The listing builds one solid part. Answer for the finished solid, in the listing's coordinates (mm). Coordinates: 2 decimals unless noted, no trailing zeros. Loops run counter-clockwise (first coordinate to the right, second up) from the corner with the lowest first, then second, coordinate; pieces in that order, holes last. Notation, with made-up numbers: (8.25, 53) - (15.25, 53) arc R28 cw to (15.25, 77) - close; hole circle Ø6 at (-23.75, 74.25). An arc over 180 degrees is marked (long way). One line per question, with ' | ' between items.
Autodesk Inventor part; units mm, degrees
ref_plane "Work Plane1" through (29, 0, 0) normal (0, -1, 0) x (1, 0, 0)
ref_plane "YZ Plane" through (0, 0, 0) normal (1, 0, 0) x (0, 1, 0)
ref_plane "XZ Plane" through (0, 0, 0) normal (0, 1, 0) x (-1, 0, 0)
sketch "Sketch1" plane through (0, 0, 0) normal (0, 0, 1) x (1, 0, 0)
  line L0 (-0.0833, 0) -> (35, 0)
  line L1 (35, 0) -> (35, 1)
  line L2 (35, 1) -> (32, 1)
  line L3 (32, 1) -> (31.6932, 1)
  line L4 (31.6932, 1) -> (0, 1)
  line L5 (0, 1) -> (0, 1.75)
  line L6 (0, 1.75) -> (-1.2, 1.75)
  line L7 (-1.2, 1.75) -> (-1.2, 0.7217)
  line L8 (-1.2, 0.7217) -> (-0.5, 0.7217)
  line L9 (-0.5, 0.7217) -> (-0.0833, 0)
  line L10 (-8.44, 0) -> (42.24, 0)
  line L11 (0, -0.35) -> (0, 2.1)
  line L12 (32, 1) -> (0, 1) construction
  dimension "d1" = 3
  dimension "d2" = 0.3068
  dimension "d3" = 1.2
  dimension "d4" = 0.7
  dimension "d5" = 60
  dimension "d6" = 2
  dimension "d7" = 2
  dimension "d8" = 1.4434
  dimension "d9" = 3.5
  dimension "d26" = 35
revolve "Body" add sketch "Sketch1" angle 360 about axis through (-0.0833, 0, 0) along (1, 0, 0)
sketch "Sketch2" plane through (-1.2, 0, 0) normal (-1, 0, 0) x (0, 0, 1)
  circle A0 centre (0, 0) radius 0.7217
  line L0 (0, -2.45) -> (0, 2.45)
  line L1 (-2.45, 0) -> (2.45, 0)
  line L2 (0.7217, 0) -> (0.3608, -0.625)
  line L3 (0.3608, -0.625) -> (-0.3608, -0.625)
  line L4 (-0.3608, -0.625) -> (-0.7217, 0)
  line L5 (-0.7217, 0) -> (-0.3608, 0.625)
  line L6 (-0.3608, 0.625) -> (0.3608, 0.625)
  line L7 (0.3608, 0.625) -> (0.7217, 0)
extrude "Slot" add sketch "Sketch2" against normal up to next contours L7 A0 | A0 L2 | L6 L0 A0 | A0 L0 L3 | L0 L6 A0 | A0 L3 L0 | L4 A0 | A0 L5
fillet "Fillet1" radius 0.8 1 edges at (-1.2, -1.75, 0)
chamfer "Chamfer1" distance 0.3067 distance2 0.3067 1 edges at (35, -1, 0) measured on face at (35, 0.3333, 0.4421)
ref_plane "Work Plane1" through (29, 0, 0) normal (0, -1, 0) x (1, 0, 0)
fillet "Fillet2" radius 0.1 1 edges at (0, -1, 0)
thread "Thread2"
equation "\"d15\" = -0.5 * SPD + 0.5 * GD"
equation "\"d16\" = GUL"
equation "\"GD\" = NND"
equation "\"NLG\" = 6"
equation "\"GEL\" = 4.5"
equation "\"KOD\" = 5.7"
equation "\"KOH\" = 1.65"
equation "\"INTI\" = 1.04"
equation "\"GAL\" = 0.61345 * PTC"
equation "\"GUL\" = 0.61345 * PTC"
equation "\"BDM\" = NND"
equation "\"SW\" = 2"
equation "\"RR\" = 1.45"
equation "\"SPD\" = NND - 1.2269 * PTC"
equation "\"R\" = 0.3"
equation "\"TOA\" = 30deg"
equation "\"GD1\" = THREADDIA - 1.2269 * PTC"
equation "\"THREADDIA\" = 3"
equation "\"PTC\" = 0.5"
equation "\"NND\" = 3"
equation "\"KOH1\" = 0.2"
equation "\"E0\" = 2.303"
properties part number "M2x35 Bolt" material "Stainless Steel"
Item 1: Find section A-A, the plane x = 3.5. Write down the section's boundary in (y, z), plus the area to 3 significant figures.
Taken from the geometry:
outline: circle Ø2 at (0, 0) | area: 3.14 mm2
Item 2: Each of these flat-tipped pins is pushed along its axis until it touches: pin 1 Ø0.6 at (x, z) = (-1, 0) entering from -Y; pin 2 Ø1 at (x, y) = (25, 0) entering from +Z; pin 3 Ø1.5 at (x, y) = (28, 1) entering from -Z. Where does it stop, or does it pass through?
Taken from the geometry:
pin 1: stops at y = -1.69 | pin 2: stops at z = 1 | pin 3: stops at z = -0.97
Item 3: The mould has two halves that part along Z. Classify faces 1 (the face through (-0.109, 0.043, -0.014)), 2 (the face through (35, 0, 0)), 3 (the face through (-0.203, 1.617, 0.67)): pulls with the +Z half, pulls with the -Z half, needs draft (parallel to the pull), parting line crosses it, or undercut.
Taken from the geometry:
face 1: undercut | face 2: needs draft | face 3: parting line crosses it
Item 4: Find the intervals of material crossed by line 1 (Z direction, x = 21, y = 0.7); line 2 (Z direction, x = 20, y = 0); line 3 (X direction, y = 1.2, z = -0.3), in increasing order. Write a range as [from, to].
Taken from the geometry:
line 1: z = [-0.71, 0.71] | line 2: z = [-1, 1] | line 3: x = [-1.15, 0]
